Work out the finished part from the listing and answer in its coordinate system (mm). A direction names the side the tool comes from. Coordinates: 2 decimals unless noted, no trailing zeros. Write each loop counter-clockwise with the first axis right and the second up, starting at its lowest first coordinate (ties: lowest second). Pieces come first, ordered by that corner, then holes. Notation, with made-up numbers: (84, -14) - (127, -14) arc R27 cw to (127, 20) - close; hole circle Ø7 at (3, 82). An arc over 180 degrees is marked (long way). Use a Markdown table: item, result. Add a question column.
(1) The part is cut by section A-A, the plane x = 12. Give the vertices of the cut face in (y, z), then the cut area to 3 significant figures.
(2) A tool of negligible diameter and unlimited length cuts with its end or side. For faces 5 (the face through (12, 12.172, -7)), 6 (the face through (12, 16, 156)), 7 (the face through (12, 14.828, -7)), from which of +Z, -Z, +X, -X, +Y, -Y can it reach the whole face along a straight path? Write none if from no direction.
(3) Find the intervals of material crossed by line 1 (Z direction, x = 12, y = 13.4); line 2 (X direction, y = 13.5, z = 116); line 3 (Z direction, x = 12, y = 22.5), in increasing order. Write a range as from..to.
(4) The part is cut by section C-C, the plane y = 9.75. Give the vertices of the cut face in (x, z), then the cut area to 3 significant figures.
(5) For a pull along Z with two mould halves and no side action, classify faces 1 (the face through (12, 4, 79)), 2 (the face through (20, 15, 79)), 3 (the face through (12, 14, 160)), 4 (the face through (3, 27, 86)) as released by +Z, released by -Z, zero draft, split by the parting line, or undercut.
(6) The part is cut by section B-B, the plane z = 85. Give the vertices of the cut face in (x, y), then the cut area to 3 significant figures.
(7) Given pin 1 Ø7 at (x, y) = (15.5, 7) entering from -Z; pin 2 Ø4 at (x, z) = (12, -10.4) entering from -Y; pin 3 Ø3 at (y, z) = (13.5, -6.5) entering from +X; pin 4 Ø8 at (x, z) = (11.5, 75.5) entering from +Y, each flat-ended and moving along its own axis, determine where each tip first touches the part or whether it passes through.
from build123d import *

# Parameters (mm, degrees)
SKETCH1_W           = 24
SKETCH1_H           = 27
BOSS_EXTRUDE1_DEPTH = 160
SHELL1_T            = -4
SKETCH2_W           = 16.655936622
SKETCH2_H           = 2.65564638
BOSS_EXTRUDE2_DEPTH = 15
SKETCH3_R           = 2.351991257
CUT_EXTRUDE1_DEPTH  = 15.82782319


with BuildPart() as part:
    # Sketch1 → Boss-Extrude1 (new body)
    with BuildSketch(Plane.XY):
        with Locations((12, 13.5)):
            Rectangle(SKETCH1_W, SKETCH1_H)
    extrude(amount=BOSS_EXTRUDE1_DEPTH)

    # Shell1
    shell1_openings = [part.faces().sort_by_distance(p)[0] for p in [
        (12, 27, 80),
    ]]
    offset(amount=SHELL1_T, openings=shell1_openings, kind=Kind.INTERSECTION)

    # Sketch2 → Boss-Extrude2 (add)
    with BuildSketch(Plane(origin=(0, 0, 0), x_dir=(-1, 0, 0), z_dir=(0, 0, -1))):
        with Locations((-12, 13.5)):
            Rectangle(SKETCH2_W, SKETCH2_H)
    extrude(amount=BOSS_EXTRUDE2_DEPTH)

    # Sketch3 → Cut-Extrude1 (cut, through all)
    with BuildSketch(Plane(origin=(0, 14.82782319, 0), x_dir=(1, 0, 0), z_dir=(0, 1, 0))):
        with Locations((12, 10.403093439)):
            Circle(SKETCH3_R)
    extrude(amount=-CUT_EXTRUDE1_DEPTH, mode=Mode.SUBTRACT)


solid = part.part
Model answer:
| question | item | result |
|---|---|---|
| 1 | outline | (0, 0) - (12.17, 0) - (12.17, -8.05) - (14.83, -8.05) - (14.83, 0) - (27, 0) - (27, 4) - (4, 4) - (4, 156) - (27, 156) - (27, 160) - (0, 160) - close; (12.17, -15) - (14.83, -15) - (14.83, -12.76) - (12.17, -12.76) - close |
| 1 | area | 851 mm^2 |
| 2 | face 5 | -Z, +X, -X, -Y |
| 2 | face 6 | +Y |
| 2 | face 7 | -Z, +X, -X, +Y |
| 3 | line 1 | -15..-12.76, -8.05..4, 156..160 |
| 3 | line 2 | 0..4, 20..24 |
| 3 | line 3 | 0..4, 156..160 |
| 4 | outline | (0, 0) - (24, 0) - (24, 160) - (0, 160) - close; hole (4, 4) - (20, 4) - (20, 156) - (4, 156) - close |
| 4 | area | 1,410 mm^2 |
| 5 | face 1 | undercut |
| 5 | face 2 | undercut |
| 5 | face 3 | released by +Z |
| 5 | face 4 | zero draft |
| 6 | outline | (0, 0) - (24, 0) - (24, 27) - (20, 27) - (20, 4) - (4, 4) - (4, 27) - (0, 27) - close |
| 6 | area | 280 mm^2 |
| 7 | pin 1 | z = 0 |
| 7 | pin 2 | through |
| 7 | pin 3 | x = 20.33 |
| 7 | pin 4 | y = 4 |
